Drawing for the job (mm, zero at the part's lowest x, y, z). Give positions to 0.01 mm unless a question says otherwise; leave off trailing zeros. Loops run counter-clockwise (first coordinate to the right, second up) from the corner with the lowest first, then second, coordinate; pieces in that order, holes last.
1) Band-saw the part on A-A on x = 44. List the corners of the cut face in (y, z) (3 decimals).
2) Band-saw the part on B-B on z = 1.6. List the corners of the cut face in (x, y) (3 decimals), then the cut area to 3 significant figures.
3) Wall check: line 1 (X direction, y = 2.5, z = 2.2); line 2 (X direction, y = 3.25, z = 0.65); line 3 (Y direction, x = 4, z = 1.35). Give the ranges that are in metal, low to high.
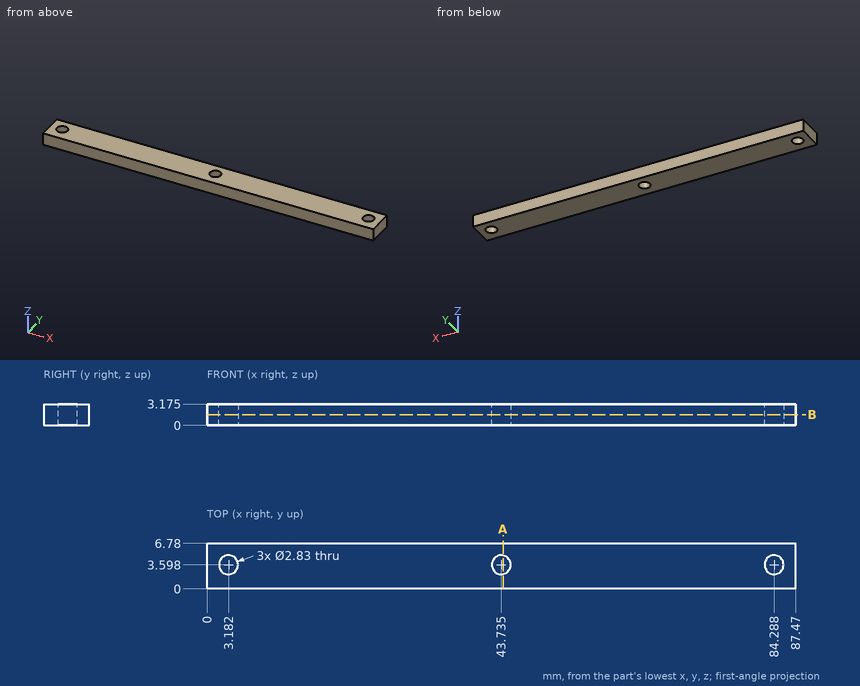
Findings below:
1. outline: (0, 0) - (2.208, 0) - (2.208, 3.175) - (0, 3.175) - close; (4.988, 0) - (6.78, 0) - (6.78, 3.175) - (4.988, 3.175) - close
2. outline: (0, 0) - (87.47, 0) - (87.47, 6.78) - (0, 6.78) - close; hole circle Ø2.83 at (3.182, 3.598); hole circle Ø2.83 at (43.735, 3.598); hole circle Ø2.83 at (84.288, 3.598)
2. area: 574 mm2
3. line 1: x = 0 to 2.29, 4.07 to 42.84, 44.63 to 83.4, 85.18 to 87.47
3. line 2: x = 0 to 1.81, 4.55 to 42.36, 45.11 to 82.92, 85.66 to 87.47
3. line 3: y = 0 to 2.44, 4.75 to 6.78
